The model under review builds one solid part; all positions refer to its coordinate system, in mm. A direction names the side the tool comes from. Give positions to 0.01 mm unless a question says otherwise; leave off trailing zeros. Order: outer loops, then holes, each group sorted by start corner. A loop starts at its lowest first (then second) coordinate and runs counter-clockwise, first axis right, second up.
```python
from build123d import *

# Parameters (mm, degrees)
F1_DEPTH       = 165.1
F2_R           = 1.524
F4_D           = 20.6375
F4_CBORE_D     = 30.1752
F4_CBORE_DEPTH = 28.448
F5_W           = 63.5
F5_H           = 330.2
F6_DEPTH       = 6.35
F8_D           = 13.49248
F8_DEPTH       = 41.2172727273
F8_TIP         = 4.0535499425


# Not quite as in the source:
# - a length typed as a fraction of an inch, garbled in the dataset ("3 / 203.2 mm" for 3/8 in), is restored


with BuildPart() as f1:
    # F0 (on Top) → F1 (new body, symmetric)
    with BuildSketch(Plane.XY):
        Polygon((95.25, 44.45), (-95.25, 44.45), (-95.25, 31.75), (-57.15, 31.75), (-57.15, -31.75), (-95.25, -31.75), (-95.25, -44.45), (95.25, -44.45), align=None)
    extrude(amount=F1_DEPTH, both=True)

    # F2
    f2_edges = [f1.edges().sort_by_distance(p)[0] for p in [
        (-57.15, 31.75, 0),
        (-57.15, -31.75, 0),
    ]]
    fillet(f2_edges, radius=F2_R)

    # F4 (through all)
    with Locations(Plane.YZ.offset(95.25)):
        with Locations((0, 107.95), (0, -107.95)):
            CounterBoreHole(F4_D / 2, F4_CBORE_D / 2, F4_CBORE_DEPTH)

    # F5 (on face) → F6 (cut)
    with BuildSketch(Plane.XZ.offset(44.45)):
        with Locations((63.5, 0)):
            Rectangle(F5_W, F5_H)
    extrude(amount=-F6_DEPTH, mode=Mode.SUBTRACT)

    # F8
    with Locations(Plane.XZ.offset(38.1)):
        with Locations((63.5, 139.7), (63.5, 0), (63.5, -139.7)):
            Hole(F8_D / 2, depth=F8_DEPTH)
            with Locations((0, 0, -(F8_DEPTH + F8_TIP / 2))):  # 118° drill point
                Cone(0, F8_D / 2, F8_TIP, mode=Mode.SUBTRACT)


solid = f1.part
```
Item 1: Take a section at B-B (x = 43.5). Give the boundary of the cut face in (y, z).
Values found:
outline: (-38.1, -165.1) - (44.45, -165.1) - (44.45, 165.1) - (-38.1, 165.1) - close; hole circle Ø20.64 at (0, -107.95); hole circle Ø20.64 at (0, 107.95)
Item 2: Take a section at C-C (z = 74.5). Give the boundary of the cut face in (x, y), and give its area (3 significant figures).
Values found:
outline: (-95.25, -44.45) - (31.75, -44.45) - (31.75, -38.1) - (95.25, -38.1) - (95.25, 44.45) - (-95.25, 44.45) - (-95.25, 31.75) - (-58.67, 31.75) arc R1.52 cw to (-57.15, 30.23) - (-57.15, -30.23) arc R1.52 cw to (-58.67, -31.75) - (-95.25, -31.75) - close
area: 14,100 mm2
Item 3: Take a section at A-A (z = 107.95). Give the boundary of the cut face in (x, y).
Values found:
outline: (-95.25, -44.45) - (31.75, -44.45) - (31.75, -38.1) - (95.25, -38.1) - (95.25, -15.09) - (66.8, -15.09) - (66.8, -10.32) - (-57.15, -10.32) - (-57.15, -30.23) arc R1.52 cw to (-58.67, -31.75) - (-95.25, -31.75) - close; (-95.25, 31.75) - (-58.67, 31.75) arc R1.52 cw to (-57.15, 30.23) - (-57.15, 10.32) - (66.8, 10.32) - (66.8, 15.09) - (95.25, 15.09) - (95.25, 44.45) - (-95.25, 44.45) - close
Item 4: Draft analysis for pull direction Z (two halves, no side actions). For faces 5 (the flat face through (-95.25, -38, 2)), 6 (the cylindrical face through (81.23, -1.96, -92.99)), state which applies: released by +Z, released by -Z, zero draft, split by the parting line, or undercut.
Values found:
face 5: zero draft
face 6: undercut
Item 5: For faces 1 (the flat face through (66.802, -4, 98)), 2 (the cylindrical face through (60.387, -17.203, 133.715)), 3 (the flat face through (56, -38.1, 2)), 4 (the flat face through (-57.15, 0, 2)), list the 3-axis set-ups (+Z, -Z, +X, -X, +Y, -Y) from which the entire face can be reached by the end or side of a thin tool; tool diameter is ignored.
Values found:
face 1: +X
face 2: -Y
face 3: +Z, -Z, +X, -Y
face 4: +Z, -Z, -X
Item 6: Clearance check with flat-ended pins moving along their axes: pin 1 Ø3 at (y, z) = (-40.5, -54.5) entering from +X; pin 2 Ø9 at (y, z) = (-4, 110.5) entering from +X; pin 3 Ø15 at (y, z) = (6, -111) entering from +X; pin 4 Ø12 at (x, z) = (63.5, 0) entering from -Y. State where each tip first meets the part, or that it passes through.
Values found:
pin 1: stops at x = 31.75
pin 2: passes through
pin 3: stops at x = 66.8
pin 4: stops at y = 3.57
Item 7: For line 1 (Z direction, x = 16, y = 0); line 2 (Z direction, x = 89, y = 0); line 3 (Z direction, x = 63, y = -20), list the stretches that pass through material, from the lowest coordinate up.
Values found:
line 1: z = -165.1 to -118.27, -97.63 to 97.63, 118.27 to 165.1
line 2: z = -165.1 to -123.04, -92.86 to 92.86, 123.04 to 165.1
line 3: z = -165.1 to -146.43, -132.97 to -6.73, 6.73 to 132.97, 146.43 to 165.1
Item 8: Take a section at D-D (y = 26). Give the boundary of the cut face in (x, z).
Values found:
outline: (-57.15, -165.1) - (95.25, -165.1) - (95.25, 165.1) - (-57.15, 165.1) - close
